```python
from build123d import *

# Parameters (mm, degrees)
F0_W     = 140
F0_H     = 160
F1_DEPTH = 15
F2_W     = 134
F2_H     = 52
F3_DEPTH = 12
F4_W     = 9
F4_H     = 100
F5_DEPTH = 7


with BuildPart() as f1:
    # F0 (on Top) → F1 (new body)
    with BuildSketch(Plane.XY):
        with Locations((14.341742, -25.477314)):
            Rectangle(F0_W, F0_H)
    extrude(amount=F1_DEPTH)

    # F2 (on face) → F3 (cut)
    with BuildSketch(Plane.XY.offset(15)):
        with Locations((14.341742, 25.522686)):
            Rectangle(F2_W, F2_H)
    extrude(amount=-F3_DEPTH, mode=Mode.SUBTRACT)

    # F4 (on face) → F5 (cut)
    with BuildSketch(Plane.XY.offset(15)):
        with Locations((-46.158258, -50.477314)):
            Rectangle(F4_W, F4_H)
        with Locations((-33.658258, -50.477314)):
            Rectangle(F4_W, F4_H)
        with Locations((-8.658258, -50.477314)):
            Rectangle(F4_W, F4_H)
        with Locations((3.841742, -50.477314)):
            Rectangle(F4_W, F4_H)
        with Locations((28.841742, -50.477314)):
            Rectangle(F4_W, F4_H)
        with Locations((41.341742, -50.477314)):
            Rectangle(F4_W, F4_H)
        with Locations((53.841742, -50.477314)):
            Rectangle(F4_W, F4_H)
        with Locations((66.341742, -50.477314)):
            Rectangle(F4_W, F4_H)
        with Locations((16.341742, -50.477314)):
            Rectangle(F4_W, F4_H)
        with Locations((-21.158258, -50.477314)):
            Rectangle(F4_W, F4_H)
    extrude(amount=-F5_DEPTH, mode=Mode.SUBTRACT)


solid = f1.part
```
Verification items for the finished model (mm, model axes). Give positions to 0.01 mm unless a question says otherwise; leave off trailing zeros. Loops run counter-clockwise (first coordinate to the right, second up) from the corner with the lowest first, then second, coordinate; pieces in that order, holes last.
1. Section check C-C, the plane x = 51.5. Enter the section's corners in (y, z), then the cut area to 3 significant figures.
2. Section check B-B, the plane z = 6. Enter the section's corners in (x, y).
3. Thickness scan on line 1 (Y direction, x = 67, z = 10.5); line 2 (Y direction, x = 73, z = 14); line 3 (X direction, y = 23, z = 11.5). Record the ranges inside material, lowest first.
4. Go/stop test with a flat-tipped pin: pin 1 Ø2.5 at (x, y) = (43.5, -63) entering from +Z. Record where the tip stops, or that it passes through.
5. Section check A-A, the plane y = 38. Enter the section's corners in (x, z).
6. Mould release check, pull along Y, two halves, no side actions. Record for faces 1 (the flat face through (-9, -100.477, 12)), 2 (the flat face through (35, -31, 15)), 3 (the flat face through (-4.158, -51, 12)): released by +Y, released by -Y, zero draft, split by the parting line, or undercut.
Geometry says:
1. outline: (-105.48, 0) - (54.52, 0) - (54.52, 15) - (51.52, 15) - (51.52, 3) - (-0.48, 3) - (-0.48, 8) - (-100.48, 8) - (-100.48, 15) - (-105.48, 15) - close
1. area: 1,080 mm2
2. outline: (-55.66, -105.48) - (84.34, -105.48) - (84.34, 54.52) - (-55.66, 54.52) - close; hole (-52.66, -0.48) - (81.34, -0.48) - (81.34, 51.52) - (-52.66, 51.52) - close
3. line 1: y = -105.48 to -100.48, 51.52 to 54.52
3. line 2: y = -105.48 to -0.48, 51.52 to 54.52
3. line 3: x = -55.66 to -52.66, 81.34 to 84.34
4. pin 1: stops at z = 8
5. outline: (-55.66, 0) - (84.34, 0) - (84.34, 15) - (81.34, 15) - (81.34, 3) - (-52.66, 3) - (-52.66, 15) - (-55.66, 15) - close
6. face 1: undercut
6. face 2: zero draft
6. face 3: undercut
